Check sheet for the modelled part. Datum: model origin and axes. Units: mm. Face numbers are marked on the shaded views. A direction names the side the tool comes from. Give positions to 0.01 mm unless a question says otherwise; leave off trailing zeros. Order: outer loops, then holes, each group sorted by start corner. A loop starts at its lowest first (then second) coordinate and runs counter-clockwise, first axis right, second up.
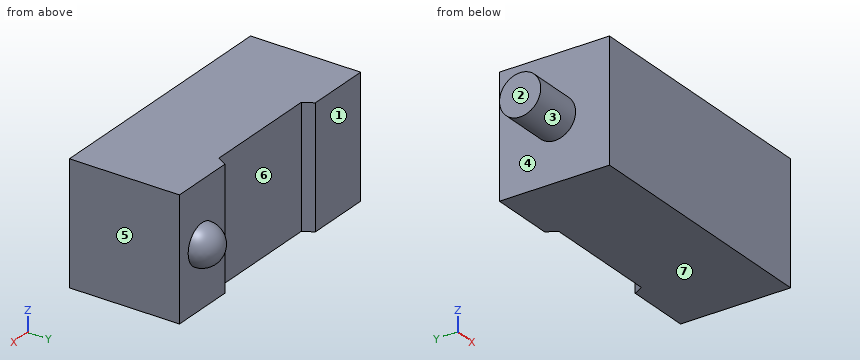
```python
from build123d import *

# Parameters (mm, degrees)
SKETCH_1_W          = 26
SKETCH_1_H          = 12
EXTRUDE_1_DEPTH     = 11
SKETCH_2_W          = 13
SKETCH_2_H          = 15
CUT_EXTRUDE_2_DEPTH = 1
CUT_EXTRUDE_2_DRAFT = -30
SKETCH_4_R          = 2.060062992
EXTRUDE_3_DEPTH     = 5


with BuildPart() as part:
    # 草图1 → 拉伸1 (new body)
    with BuildSketch(Plane(origin=(0, 0, 0), x_dir=(1, 0, 0), z_dir=(0, 1, 0))):
        Rectangle(SKETCH_1_W, SKETCH_1_H)
    extrude(amount=EXTRUDE_1_DEPTH)


with BuildPart() as cut_extrude_2_tool:
    # 草图2 → 拉伸2 (with draft: the straight prism first)
    with BuildSketch(Plane(origin=(0, 11, 0), x_dir=(1, 0, 0), z_dir=(0, 1, 0))):
        Rectangle(SKETCH_2_W, SKETCH_2_H)
    extrude(amount=-CUT_EXTRUDE_2_DEPTH)
    # 拉伸2: the draft: its side faces are tilted about the plane it starts from
    cut_extrude_2_sides = [cut_extrude_2_tool.faces().sort_by_distance(p)[0] for p in [
        (0, 10.5, 7.5),
        (6.5, 10.5, 0),
        (0, 10.5, -7.5),
        (-6.5, 10.5, 0),
    ]]
    draft(cut_extrude_2_sides, Plane(origin=(0, 11, 0), x_dir=(1, 0, 0), z_dir=(0, 1, 0)), CUT_EXTRUDE_2_DRAFT)


with BuildPart() as part_1:
    add(part.part)

    # 拉伸2: cut by cut_extrude_2_tool
    add(cut_extrude_2_tool.part, mode=Mode.SUBTRACT)

    # 草图3 → 旋转1 (revolve)
    with BuildSketch(Plane.XY):
        with BuildLine():
            Line((9.75, 13), (9.75, 9))
            ThreePointArc((9.75, 9), (11.75, 11), (9.75, 13))
        make_face()
    revolve(axis=Axis((9.75, 13, 0), (0, -1, 0)))

    # 草图4 → 拉伸3 (add)
    with BuildSketch(Plane.ZY.offset(13)):
        with Locations(Location((0, 5.445496221, 0), (0, 0, 180))):
            Circle(SKETCH_4_R)
    extrude(amount=EXTRUDE_3_DEPTH)


solid = part_1.part
```
(1) Gauge pin test, flat ends, axial feed: pin 1 Ø2 at (x, z) = (-11, -1) entering from +Y; pin 2 Ø7 at (x, z) = (11, -0.5) entering from +Y. Record the tip position at first contact, or that the pin passes through.
Response values:
pin 1: stops at y = 11
pin 2: stops at y = 13
(2) Cross-section at C-C on y = 8.75. Enter the section's corners in (x, z).
Response values:
outline: (-13, -6) - (13, -6) - (13, 6) - (-13, 6) - close
(3) Material ranges on L1, parallel to X at y = 10.5, z = -2; L2, parallel to Y at x = -8, z = -1.5; L3, parallel to X at y = 1.25, z = 4.75, recorded low to high.
Response values:
L1: x = -13 to -6.21, 6.21 to 13
L2: y = 0 to 11
L3: x = -13 to 13
(4) Set-up check for the marked faces 1, 2 and 3: record each of +Z, -Z, +X, -X, +Y, -Y from which the full face is reachable in a straight line by a thin tool's end or side.
Response values:
face 1: +Z, -Z, -X, +Y
face 2: +Z, -Z, -X, +Y, -Y
face 3: -X
(5) Cross-section at A-A on z = 0. Enter the section's corners in (x, y).
Response values:
outline: (-18, 3.39) - (-13, 3.39) - (-13, 0) - (13, 0) - (13, 11) - (11.75, 11) arc R2 ccw to (7.75, 11) - (6.5, 11) - (5.92, 10) - (-5.92, 10) - (-6.5, 11) - (-13, 11) - (-13, 7.51) - (-18, 7.51) - close
(6) Release check for a two-part mould opening along X. For the marked faces 4, 5, 6 and 7 record: released by +X, released by -X, zero draft, split by the parting line, or undercut.
Response values:
face 4: released by -X
face 5: released by +X
face 6: undercut
face 7: zero draft
(7) Cross-section at D-D on z = 4. Enter the section's corners in (x, y).
Response values:
outline: (-13, 0) - (13, 0) - (13, 11) - (6.5, 11) - (5.92, 10) - (-5.92, 10) - (-6.5, 11) - (-13, 11) - close
(8) Cross-section at B-B on x = -2.5. Enter the section's corners in (y, z).
Response values:
outline: (0, -6) - (10, -6) - (10, 6) - (0, 6) - close
